Geometry: final body of the model. Coordinates: model frame, mm. Face numbers are marked on the shaded views. A direction names the side the tool comes from. Round coordinates to 2 decimals unless told otherwise and drop trailing zeros. Loops run counter-clockwise (first coordinate to the right, second up) from the corner with the lowest first, then second, coordinate; pieces in that order, holes last. Notation, with made-up numbers: (-39, 5) -> (-16, 5) arc R26 cw to (-16, 27) -> close; hole circle Ø6 at (70.25, 69). An arc over 180 degrees is marked (long way). Answer in a Markdown table with one row per item.
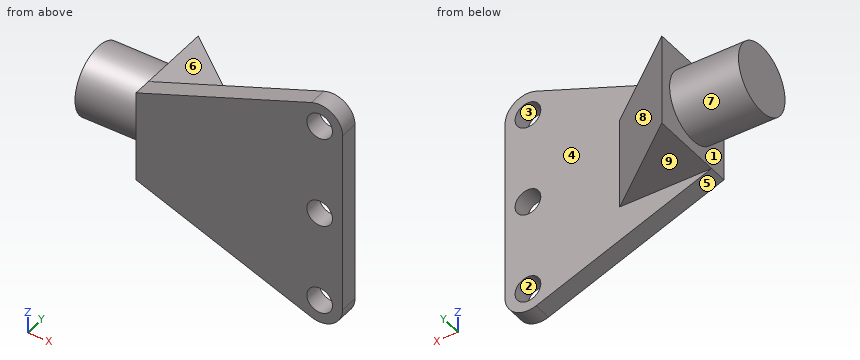
```python
from build123d import *

# Parameters (mm, degrees)
SKETCH2_W           = 25.4
SKETCH2_H           = 25.4
BOSS_EXTRUDE1_DEPTH = 25.4
BOSS_EXTRUDE2_DEPTH = 5.08
SKETCH5_R           = 3.556
CUT_EXTRUDE1_DEPTH  = 5.08
SKETCH6_R           = 3.556
CUT_EXTRUDE2_DEPTH  = 5.08
CUT_EXTRUDE3_DEPTH  = 25.4
SKETCH10_R          = 9.525
BOSS_EXTRUDE3_DEPTH = 19.05
CUT_EXTRUDE4_REACH  = 82.822
SKETCH12_R          = 3.556


with BuildPart() as part:
    # Sketch2 → Boss-Extrude1 (new body)
    with BuildSketch(Plane(origin=(0, 0, 0), x_dir=(1, 0, 0), z_dir=(0, 1, 0))):
        with Locations((-38.1, 0)):
            Rectangle(SKETCH2_W, SKETCH2_H)
    extrude(amount=BOSS_EXTRUDE1_DEPTH)

    # Sketch8 → Cut-Extrude3 (cut)
    with BuildSketch(Plane(origin=(0, 0, -12.7), x_dir=(-1, 0, 0), z_dir=(0, 0, -1))):
        Polygon((50.8, 25.4), (25.4, 5.08), (25.4, 25.4), align=None)
    extrude(amount=-CUT_EXTRUDE3_DEPTH, mode=Mode.SUBTRACT)



with BuildPart() as body_2:
    # Sketch4 → Boss-Extrude2 (new body)
    with BuildSketch(Plane(origin=(0, 0, 0), x_dir=(1, 0, 0), z_dir=(0, 1, 0))):
        with BuildLine():
            Line((-50.8, -12.7), (-2.275658989, -31.327921356))
            ThreePointArc((-2.275658989, -31.327921356), (3.596462869, -30.633003943), (6.349714595, -25.4))
            Line((6.349714595, -25.4), (6.35, 25.4))
            ThreePointArc((6.35, 25.4), (3.596610154, 30.633249029), (-2.275793827, 31.328175306))
            Line((-2.275793827, 31.328175306), (-50.8, 12.7))
            Line((-50.8, 12.7), (-50.8, -12.7))
        make_face()
    extrude(amount=BOSS_EXTRUDE2_DEPTH)

    # Sketch5 → Cut-Extrude1 (cut)
    with BuildSketch(Plane(origin=(0, 0, 0), x_dir=(1, 0, 0), z_dir=(0, 1, 0))):
        with Locations(Location((0, -25.4, 0), (0, 0, 90))):
            Circle(SKETCH5_R)
    extrude(amount=CUT_EXTRUDE1_DEPTH, mode=Mode.SUBTRACT)

    # Sketch6 → Cut-Extrude2 (cut)
    with BuildSketch(Plane(origin=(0, 0, 0), x_dir=(1, 0, 0), z_dir=(0, 1, 0))):
        with Locations(Location((0, 25.4, 0), (0, 0, 90))):
            Circle(SKETCH6_R)
    extrude(amount=CUT_EXTRUDE2_DEPTH, mode=Mode.SUBTRACT)


with BuildPart() as part_1:
    add(part.part)

    add(body_2.part)  # Boss-Extrude3 merges body 2
    # Sketch10 → Boss-Extrude3 (add)
    with BuildSketch(Plane.ZY.offset(50.8)):
        with Locations(Location((0, 12.7, 0), (0, 0, 180))):
            Circle(SKETCH10_R)
    extrude(amount=BOSS_EXTRUDE3_DEPTH)

    # Sketch12 → Cut-Extrude4 (cut, up to next)
    with BuildSketch(Plane(origin=(0, 0, 0), x_dir=(1, 0, 0), z_dir=(0, 1, 0)), mode=Mode.PRIVATE) as cut_extrude4_sk1:
        with Locations(Location((0, 0, 0), (0, 0, 90))):
            Circle(SKETCH12_R)
    cut_extrude4_tool1 = extrude(cut_extrude4_sk1.sketch, amount=CUT_EXTRUDE4_REACH, mode=Mode.PRIVATE) & part_1.part
    add(cut_extrude4_tool1.solids().sort_by_distance((0, 0, 0))[0], mode=Mode.SUBTRACT)


solid = part_1.part
```
Item 1: Set-up query: the marked faces 5, 6, 7, 8 and 9. Return all of +Z, -Z, +X, -X, +Y, -Y with unobstructed straight access to the full face (end or side cutting, diameter ignored); none if empty.
Ans:
| item | result |
|---|---|
| face 5 | -Z, -X, +Y, -Y |
| face 6 | +Z, +X, -X, +Y |
| face 7 | -X |
| face 8 | +Z, -Z, +X, +Y |
| face 9 | -Z, +X, -X, +Y |
Item 2: Mould query, pull axis X, two halves, no side actions, for the marked faces 1, 2, 3 and 4. Classes: released by +X, released by -X, zero draft, split by the parting line, or undercut.
Ans:
| item | result |
|---|---|
| face 1 | released by -X |
| face 2 | undercut |
| face 3 | undercut |
| face 4 | zero draft |
Item 3: Section query A-A, the plane x = 0. Output: boundary loops of the cut face in (y, z), and give its area (3 significant figures).
Ans:
| item | result |
|---|---|
| outline | (0, -31.75) -> (5.08, -31.75) -> (5.08, -28.96) -> (0, -28.96) -> close; (0, -21.84) -> (5.08, -21.84) -> (5.08, -3.56) -> (0, -3.56) -> close; (0, 3.56) -> (5.08, 3.56) -> (5.08, 21.84) -> (0, 21.84) -> close; (0, 28.96) -> (5.08, 28.96) -> (5.08, 31.75) -> (0, 31.75) -> close |
| area | 214 mm2 |
Item 4: Section query C-C, the plane y = 19.25. Output: boundary loops of the cut face in (x, z).
Ans:
| item | result |
|---|---|
| outline | (-69.85, -6.92) -> (-50.8, -6.92) -> (-50.8, -12.7) -> (-43.11, -12.7) -> (-43.11, 12.7) -> (-50.8, 12.7) -> (-50.8, 6.92) -> (-69.85, 6.92) -> close |
Item 5: Section query B-B, the plane z = 0. Output: boundary loops of the cut face in (x, y) (3 decimals).
Ans:
| item | result |
|---|---|
| outline | (-69.85, 3.175) -> (-50.8, 3.175) -> (-50.8, 0) -> (-3.556, 0) -> (-3.556, 5.08) -> (-25.4, 5.08) -> (-50.8, 25.4) -> (-50.8, 22.225) -> (-69.85, 22.225) -> close; (3.556, 0) -> (6.35, 0) -> (6.35, 5.08) -> (3.556, 5.08) -> close |
Item 6: Ray query, L1, parallel to X at y = 2.4, z = 0; L2, parallel to X at y = 3.5, z = 0; L3, parallel to Y at x = -20, z = -0.5. Return the intervals inside material, ascending.
Ans:
| item | result |
|---|---|
| L1 | -50.8 to -3.56, 3.56 to 6.35 |
| L2 | -69.85 to -3.56, 3.56 to 6.35 |
| L3 | 0 to 5.08 |
Item 7: Section query D-D, the plane z = -8.5. Output: boundary loops of the cut face in (x, y).
Ans:
| item | result |
|---|---|
| outline | (-69.85, 8.4) -> (-50.8, 8.4) -> (-50.8, 0) -> (6.35, 0) -> (6.35, 5.08) -> (-25.4, 5.08) -> (-50.8, 25.4) -> (-50.8, 17) -> (-69.85, 17) -> close |
Item 8: First-contact query: P1, Ø4, axis at x = -50, z = -14.5, coming from the -Y side; P2, Ø2, axis at y = 21, z = 0, coming from the +X side; P3, Ø1, axis at x = -45, y = 21, coming from the -Z side; P4, Ø3, axis at y = 8, z = -0.5, coming from the +X side (3 decimals). Flat tips, straight axial feed; report the tip coordinate or a pass-through.
Ans:
| item | result |
|---|---|
| P1 | y = 0 |
| P2 | x = -44.05 |
| P3 | z = -12.7 |
| P4 | x = -27.175 |
